from build123d import *

# Parameters (mm, degrees)
F0_W     = 82.09557
F0_H     = 137.457938
F1_DEPTH = 56.134
F2_R     = 5.08
F3_W     = 55.741566
F3_H     = 31.093935
F5_DEPTH = 129.286
F4_R     = 33.290636
F6_DEPTH = 42.672


with BuildPart() as f1:
    # F0 (on Front) → F1 (new body)
    with BuildSketch(Plane.XZ):
        Rectangle(F0_W, F0_H)
    extrude(amount=F1_DEPTH)

    # F2
    f2_edges = [f1.edges().sort_by_distance(p)[0] for p in [
        (0, -56.134, 68.728969),
        (41.047785, -28.067, 68.728969),
        (0, 0, 68.728969),
        (-41.047785, -28.067, 68.728969),
        (41.047785, -56.134, 0),
        (-41.047785, -56.134, 0),
        (0, -56.134, -68.728969),
        (41.047785, -28.067, -68.728969),
        (0, 0, -68.728969),
        (-41.047785, -28.067, -68.728969),
        (41.047785, 0, 0),
        (-41.047785, 0, 0),
    ]]
    fillet(f2_edges, radius=F2_R)

    # F3 (on face) → F5 (cut)
    with BuildSketch(Plane.XY.offset(68.728969)):
        with Locations((1.232381, -28.344775)):
            Rectangle(F3_W, F3_H)
    extrude(amount=-F5_DEPTH, mode=Mode.SUBTRACT)

    # F4 (on face) → F6 (cut)
    with BuildSketch(Plane.XZ.offset(56.134)):
        Circle(F4_R)
    extrude(amount=-F6_DEPTH, mode=Mode.SUBTRACT)


solid = f1.part
Work out the finished part from the listing and answer in its coordinate system (mm). A direction names the side the tool comes from. Round coordinates to 2 decimals unless told otherwise and drop trailing zeros. Order: outer loops, then holes, each group sorted by start corner. A loop starts at its lowest first (then second) coordinate and runs counter-clockwise, first axis right, second up. Notation, with made-up numbers: M 7,57 L 39,57 A19 ccw 39,82 Z; hole C 13.25,-23 d6. An arc over 180 degrees is marked long. One line per item, written item: value.
Q1. Flat-ended cylindrical pins translate along their axes: pin 1 (10 mm diameter, centred on x = -12.5, z = 2.5, fed in from -Y); pin 2 (2 mm diameter, centred on x = -29.5, z = 2.5, fed in from -Y); pin 3 (9.5 mm diameter, centred on x = -9.5, y = -29, fed in from +Z); pin 4 (6 mm diameter, centred on x = -18.5, y = -43, fed in from +Z). Find the tip coordinate at first contact, or state that the pin passes through.
Derived:
pin 1: y = -12.8
pin 2: y = -13.46
pin 3: z = -60.56
pin 4: z = 68.73
Q2. Determine the mould class of faces 1 (the face through (-29, -13.462, 0)), 2 (the face through (39.5, -28.4, -67.3)), 3 (the face through (29.103, -29, 19)), 4 (the face through (-39.6, -28.4, 67.2)) for opening direction X: released by +X, released by -X, zero draft, split by the parting line, or undercut.
Derived:
face 1: undercut
face 2: released by +X
face 3: undercut
face 4: released by -X
Q3. Straight lines are drawn through the part: line 1 (X direction, y = -41, z = -29); line 2 (Y direction, x = -21.5, z = -60.5); line 3 (Z direction, x = 0, y = -50). For each, find the intervals that lie inside material, in ascending order.
Derived:
line 1: -41.05 to -26.64, 29.1 to 41.05
line 2: -56.13 to -43.89, -12.8 to 0
line 3: -68.73 to -33.29, 33.29 to 68.73
Q4. Find section D-D on z = 0. Write down the section's boundary in (x, y).
Derived:
outline: M -41.05,-51.05 A5.08 ccw -35.97,-56.13 L -33.29,-56.13 L -33.29,-13.46 L -26.64,-13.46 L -26.64,-12.8 L 29.1,-12.8 L 29.1,-13.46 L 33.29,-13.46 L 33.29,-56.13 L 35.97,-56.13 A5.08 ccw 41.05,-51.05 L 41.05,-5.08 A5.08 ccw 35.97,0 L -35.97,0 A5.08 ccw -41.05,-5.08 Z
Q5. For faces 5 (the face through (-26.638, -29, 34)), 6 (the face through (-1, 0, 1)), determine the directions among +Z, -Z, +X, -X, +Y, -Y from which every point of the face is accessible in a straight line to the end or side of a thin tool.
Derived:
face 5: +Z
face 6: +Z, -Z, +X, -X, +Y
Q6. Find section C-C on y = -37. Write down the section's boundary in (x, z).
Derived:
outline: M -41.05,-63.65 A5.08 ccw -35.97,-68.73 L 35.97,-68.73 A5.08 ccw 41.05,-63.65 L 41.05,63.65 A5.08 ccw 35.97,68.73 L 29.1,68.73 L 29.1,16.16 A33.29 cw 29.1,-16.16 L 29.1,-60.56 L -26.64,-60.56 L -26.64,-19.97 A33.29 cw -26.64,19.97 L -26.64,68.73 L -35.97,68.73 A5.08 ccw -41.05,63.65 Z
Q7. Find section A-A on x = 0. Write down the section's boundary in (y, z).
Derived:
outline: M -56.13,-63.65 A5.08 ccw -51.05,-68.73 L -5.08,-68.73 A5.08 ccw 0,-63.65 L 0,63.65 A5.08 ccw -5.08,68.73 L -12.8,68.73 L -12.8,-60.56 L -43.89,-60.56 L -43.89,-33.29 L -56.13,-33.29 Z; M -56.13,33.29 L -43.89,33.29 L -43.89,68.73 L -51.05,68.73 A5.08 ccw -56.13,63.65 Z
Q8. Find section B-B on z = 42. Write down the section's boundary in (x, y), then the cut area to 3 significant figures.
Derived:
outline: M -41.05,-51.05 A5.08 ccw -35.97,-56.13 L 35.97,-56.13 A5.08 ccw 41.05,-51.05 L 41.05,-5.08 A5.08 ccw 35.97,0 L -35.97,0 A5.08 ccw -41.05,-5.08 Z; hole M -26.64,-43.89 L 29.1,-43.89 L 29.1,-12.8 L -26.64,-12.8 Z
area: 2,850 mm²
